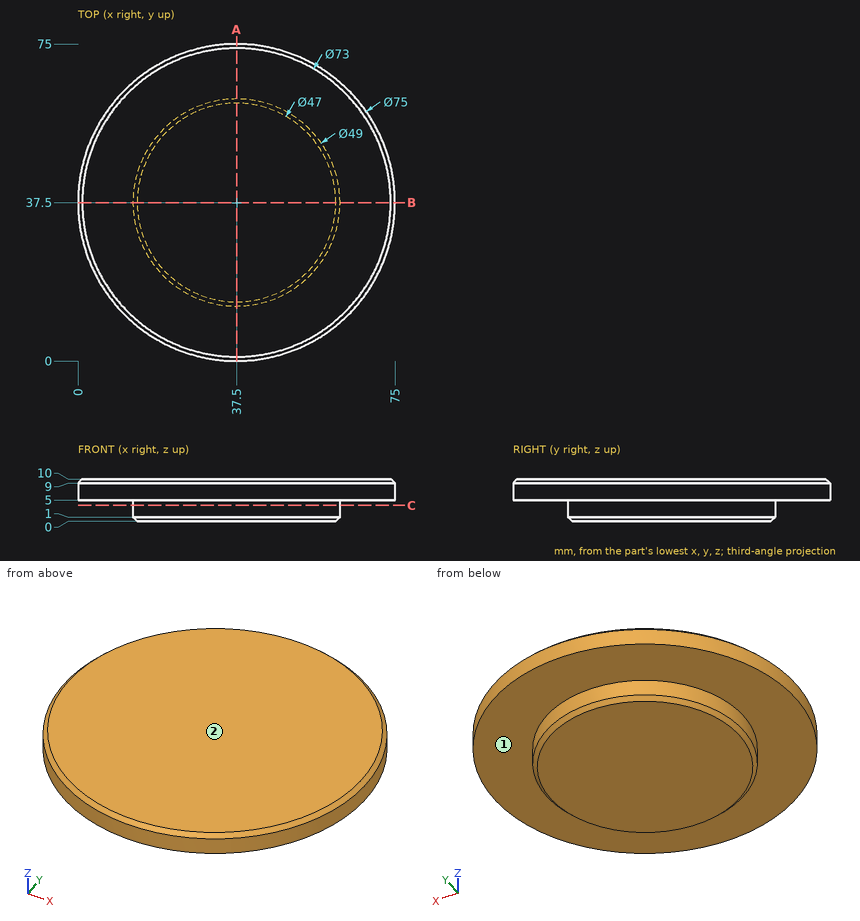
Here's the drawing with two shaded views (mm, measured from the low corner). I have some questions. A direction names the side the tool comes from. Round coordinates to 2 decimals unless told otherwise and drop trailing zeros. Loops run counter-clockwise (first coordinate to the right, second up) from the corner with the lowest first, then second, coordinate; pieces in that order, holes last.
1. If I drill on probe 1 along Z at (x, y) = (67, 49.5); probe 2 along X at (y, z) = (24, 3); probe 3 along Y at (x, z) = (3.5, 8), over which ranges is the centre line in solid material (lowest first)?
Answers:
probe 1: z = 5 to 10
probe 2: x = 17.05 to 57.95
probe 3: y = 21.68 to 53.32
2. Suppose I cut it at A-A, the plane x = 37.5. Please give me the cut outline in (y, z).
Answers:
outline: (0, 5) - (13, 5) - (13, 1) - (14, 0) - (61, 0) - (62, 1) - (62, 5) - (75, 5) - (75, 9) - (74, 10) - (1, 10) - (0, 9) - close
3. Will these pins go through, and if not, where does the flat tip stop? pin 1 (1 mm diameter, centred on x = 52, z = 2.5, fed in from -Y); pin 2 (4 mm diameter, centred on x = 32, z = 2.5, fed in from -Y); pin 3 (1.5 mm diameter, centred on y = 66.5, z = 4.5, fed in from +X).
Answers:
pin 1: stops at y = 17.39
pin 2: stops at y = 13.25
pin 3: stops at x = 61.94
4. For the marked faces 1 and 2, which set-ups out of +Z, -Z, +X, -X, +Y, -Y let a thin tool reach every point of the face, with its end or its side?
Answers:
face 1: -Z
face 2: +Z, +X, -X, +Y, -Y
5. Suppose I cut it at C-C, the plane z = 3.75. Please give me the cut outline in (x, y), and give its area (3 significant figures).
Answers:
outline: circle Ø49 at (37.5, 37.5)
area: 1,890 mm2
